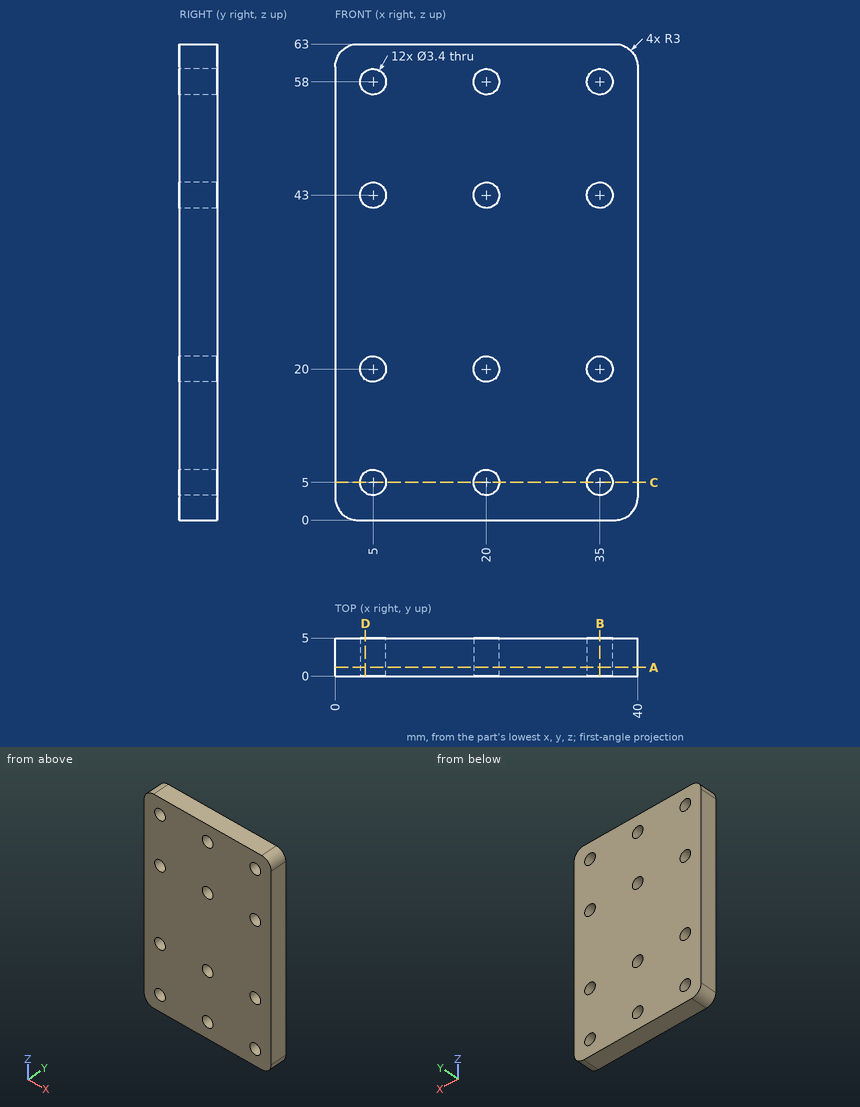
Geometry: see drawing. Coordinates: mm, zero at the bounding-box minimum. Round coordinates to 2 decimals unless told otherwise and drop trailing zeros. Loops run counter-clockwise (first coordinate to the right, second up) from the corner with the lowest first, then second, coordinate; pieces in that order, holes last. Notation, with made-up numbers: (38, -10.75) - (80, -10.75) arc R19 cw to (80, 13.25) - close; hole circle Ø11 at (68, 68.25). An arc over 180 degrees is marked (long way). One line per item, written item: value. Start each with the question number.
(1) Section D-D, the plane x = 4. Return loops of the section in (y, z).
(2) Section C-C, the plane z = 5. Return loops of the section in (x, y), plus the area to 3 significant figures.
(3) Section B-B, the plane x = 35. Return loops of the section in (y, z), plus the area to 3 significant figures.
(4) Section A-A, the plane y = 1.15. Count the separate pieces of the cut face and the enclosed holes in it, plus the area to 3 significant figures.
(5) Ray query, line 1 (Z direction, x = 35, y = 3.8); line 2 (X direction, y = 1.85, z = 5); line 3 (Z direction, x = 35.5, y = 3.1). Return the intervals inside material, ascending. Write a range as [from, to].
(6) Contact query for a flat-ended pin moving along its axis: P1, Ø2, axis at x = 20, z = 20, coming from the +Y side. Output: stop coordinate, or through.
Results below:
1. outline: (0, 0) - (5, 0) - (5, 3.63) - (0, 3.63) - close; (0, 6.37) - (5, 6.37) - (5, 18.63) - (0, 18.63) - close; (0, 21.37) - (5, 21.37) - (5, 41.63) - (0, 41.63) - close; (0, 44.37) - (5, 44.37) - (5, 56.63) - (0, 56.63) - close; (0, 59.37) - (5, 59.37) - (5, 63) - (0, 63) - close
2. outline: (0, 0) - (3.3, 0) - (3.3, 5) - (0, 5) - close; (6.7, 0) - (18.3, 0) - (18.3, 5) - (6.7, 5) - close; (21.7, 0) - (33.3, 0) - (33.3, 5) - (21.7, 5) - close; (36.7, 0) - (40, 0) - (40, 5) - (36.7, 5) - close
2. area: 149 mm^2
3. outline: (0, 0) - (5, 0) - (5, 3.3) - (0, 3.3) - close; (0, 6.7) - (5, 6.7) - (5, 18.3) - (0, 18.3) - close; (0, 21.7) - (5, 21.7) - (5, 41.3) - (0, 41.3) - close; (0, 44.7) - (5, 44.7) - (5, 56.3) - (0, 56.3) - close; (0, 59.7) - (5, 59.7) - (5, 63) - (0, 63) - close
3. area: 247 mm^2
4. separate pieces: 1
4. enclosed holes: 12
4. area: 2,400 mm^2
5. line 1: [0, 3.3], [6.7, 18.3], [21.7, 41.3], [44.7, 56.3], [59.7, 63]
5. line 2: [0, 3.3], [6.7, 18.3], [21.7, 33.3], [36.7, 40]
5. line 3: [0, 3.38], [6.62, 18.38], [21.62, 41.38], [44.62, 56.38], [59.62, 63]
6. P1: through
